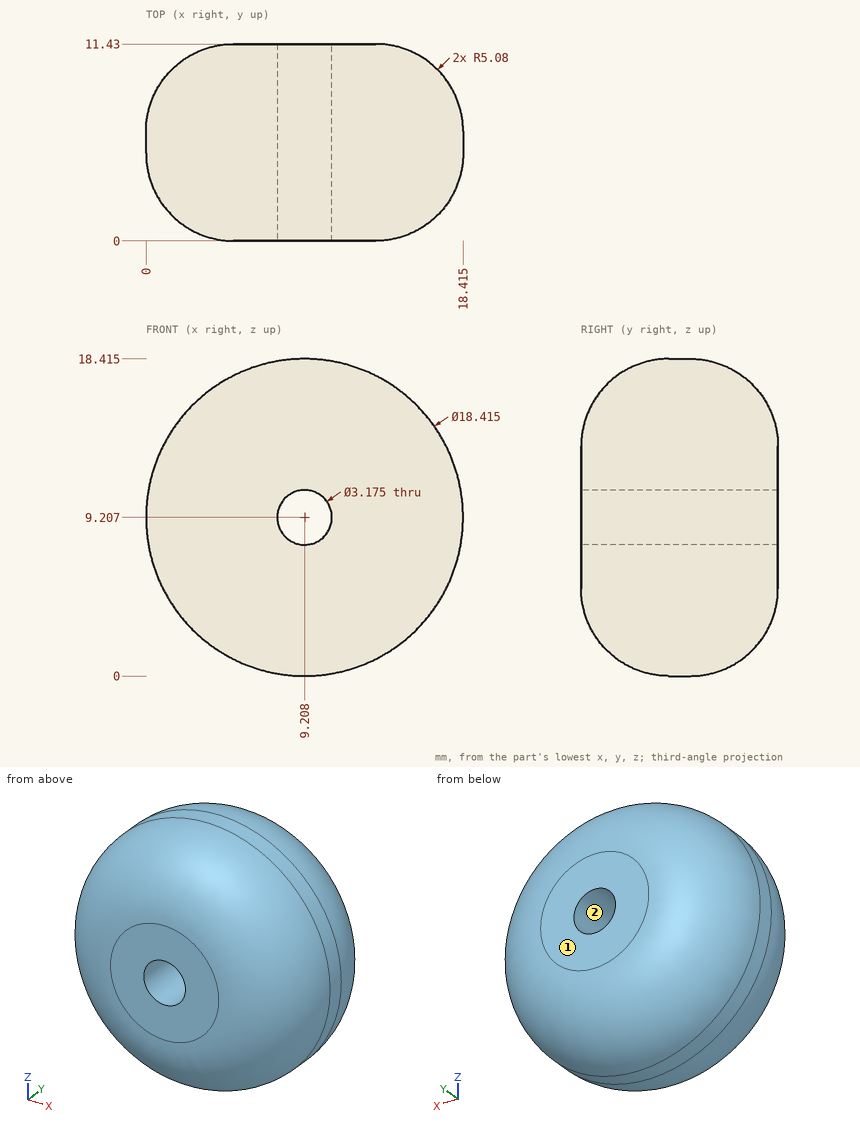
Source: three-view drawing plus pictorial views. Frame: mm from the lowest corner of the part. Round coordinates to 2 decimals unless told otherwise and drop trailing zeros. Put each result on its own line as item: value.
(1) Ray query, line 1 (Y direction, x = 13.5, z = 9); line 2 (Z direction, x = 2.25, y = 6) (1 decimal); line 3 (X direction, y = 6.5, z = 4.75) (1 decimal). Return the intervals inside material, ascending. Write a range as [from, to].
Solutions:
line 1: [0, 11.43]
line 2: [3.2, 15.2]
line 3: [1.2, 17.3]
(2) Pull-direction query (Z, two-part tool) for the marked faces 1 and 2; classes: released by +Z, released by -Z, zero draft, split by the parting line, or undercut.
Solutions:
face 1: zero draft
face 2: undercut
(3) First-contact query: pin 1 (4 mm diameter, centred on x = 9.5, y = 9, fed in from +Z); pin 2 (1.5 mm diameter, centred on x = 8.5, z = 11, fed in from -Y); pin 3 (2 mm diameter, centred on y = 2.5, z = 7, fed in from +X); pin 4 (1 mm diameter, centred on x = 14.5, y = 9, fed in from -Z) (1 decimal). Flat tips, straight axial feed; report the tip coordinate or a pass-through.
Solutions:
pin 1: z = 18.37
pin 2: y = 0
pin 3: x = 17.95
pin 4: z = 2.1
